from build123d import *

# Parameters (mm, degrees)
SKETCH_1_R      = 6
SKETCH_1_R_2    = 1.5
EXTRUDE_1_DEPTH = 4


with BuildPart() as part:
    # 草图1 → 凸台-拉伸1 (new body)
    with BuildSketch(Plane.XY):
        Circle(SKETCH_1_R)
        Circle(SKETCH_1_R_2, mode=Mode.SUBTRACT)
    extrude(amount=EXTRUDE_1_DEPTH)

    # 草图2 → 切除-旋转1 (revolve, cut)
    with BuildSketch(Plane(origin=(0, 0, 0), x_dir=(0, 0, -1), z_dir=(1, 0, 0)), mode=Mode.PRIVATE) as cut_revolve_1_sk:
        Polygon((-3.4, 6), (-2, 4.9), (-0.6, 6), align=None)
    revolve(cut_revolve_1_sk.sketch.rotate(Axis((0, 0, 0), (0, 0, 1)), 90), axis=Axis((0, 0, 0), (0, 0, 1)), mode=Mode.SUBTRACT)


solid = part.part
The listing builds one solid part. Answer for the finished solid, in the listing's coordinates (mm). Coordinates: 2 decimals unless noted, no trailing zeros. Loops run counter-clockwise (first coordinate to the right, second up) from the corner with the lowest first, then second, coordinate; pieces in that order, holes last. Notation, with made-up numbers: (88.25, 58) -> (110.25, 58) arc R20 ccw to (110.25, 68) -> close; hole circle Ø9 at (-20, -36.75). An arc over 180 degrees is marked (long way). Answer in a Markdown table with one row per item. Add a question column.
1. The part is cut by section A-A, the plane x = 0. Write down the section's boundary in (y, z), then the cut area to 3 significant figures.
2. Consider line 1 (Y direction, x = -1, z = 3.6); line 2 (X direction, y = -0.75, z = 2.7); line 3 (Y direction, x = 0.5, z = 3.35). Determine where each line is inside the solid, lowest interval first. Write a range as [from, to].
3. Determine the mould class of faces 1 (the flat face through (1.2, -1.2, 4)), 2 (the flat face through (1.2, -1.2, 0)), 3 (the cylindrical face through (-5.994, 0.264, 3.696)) for opening direction Z: +Z half, -Z half, draft (parallel to the pull), parting line (faces both ways), or undercut.
4. Flat-ended cylindrical pins translate along their axes: P1, Ø2.5, axis at x = 0, y = 0, coming from the +Z side; P2, Ø2, axis at x = -4, y = -4.5, coming from the -Z side. Find the tip coordinate at first contact, or state that the pin passes through.
5. The part is cut by section C-C, the plane z = 3.6. Write down the section's boundary in (x, y), then the cut area to 3 significant figures.
6. The part is cut by section D-D, the plane z = 2.8. Write down the section's boundary in (x, y).
Answer below:
| question | item | result |
|---|---|---|
| 1 | outline | (-6, 0) -> (-1.5, 0) -> (-1.5, 4) -> (-6, 4) -> (-6, 3.4) -> (-4.9, 2) -> (-6, 0.6) -> close; (1.5, 0) -> (6, 0) -> (6, 0.6) -> (4.9, 2) -> (6, 3.4) -> (6, 4) -> (1.5, 4) -> close |
| 1 | area | 32.9 mm2 |
| 2 | line 1 | [-5.92, -1.12], [1.12, 5.92] |
| 2 | line 2 | [-5.4, -1.3], [1.3, 5.4] |
| 2 | line 3 | [-5.94, -1.41], [1.41, 5.94] |
| 3 | face 1 | +Z half |
| 3 | face 2 | -Z half |
| 3 | face 3 | draft |
| 4 | P1 | through |
| 4 | P2 | z = 0 |
| 5 | outline | circle Ø12 at (0, 0); hole circle Ø3 at (0, 0) |
| 5 | area | 106 mm2 |
| 6 | outline | circle Ø11.06 at (0, 0); hole circle Ø3 at (0, 0) |
